from build123d import *

# Parameters (mm, degrees)
SKETCH1_W           = 10
SKETCH1_H           = 26.532998322
SKETCH1_R           = 2.25
SKETCH1_R_2         = 1.75
BOSS_EXTRUDE1_DEPTH = 4
SKETCH6_W           = 12
SKETCH6_H           = 6
BOSS_EXTRUDE3_DEPTH = 3.5
FILLET1_R           = 2
FILLET2_R           = 2
FILLET3_R           = 0.5
FILLET4_R           = 2


with BuildPart() as part:
    # Sketch1 → Boss-Extrude1 (new body)
    with BuildSketch(Plane.XY):
        with Locations((38, 0)):
            Rectangle(SKETCH1_W, SKETCH1_H)
        with Locations((38, 0)):
            Circle(SKETCH1_R, mode=Mode.SUBTRACT)
        with Locations((38, 10)):
            Circle(SKETCH1_R_2, mode=Mode.SUBTRACT)
        with Locations(Location((38, -10, 0), (0, 0, 180))):
            Circle(SKETCH1_R_2, mode=Mode.SUBTRACT)
    extrude(amount=BOSS_EXTRUDE1_DEPTH)

    # Sketch6 → Boss-Extrude3 (add)
    with BuildSketch(Plane.XY):
        with Locations((49, 0)):
            Rectangle(SKETCH6_W, SKETCH6_H)
    extrude(amount=BOSS_EXTRUDE3_DEPTH)

    # Fillet1
    fillet1_edges = [part.edges().sort_by_distance(p)[0] for p in [
        (55, -3, 1.75),
        (55, 3, 1.75),
    ]]
    fillet(fillet1_edges, radius=FILLET1_R)

    # Fillet2
    fillet2_edges = [part.edges().sort_by_distance(p)[0] for p in [
        (43, 3, 1.75),
        (43, -3, 1.75),
    ]]
    fillet(fillet2_edges, radius=FILLET2_R)

    # Fillet3
    fillet3_edges = [part.edges().sort_by_distance(p)[0] for p in [
        (43, 0, 3.5),
    ]]
    fillet(fillet3_edges, radius=FILLET3_R - 0.0001)  # a hair under: the kernel refuses the full size

    # Fillet4
    fillet4_edges = [part.edges().sort_by_distance(p)[0] for p in [
        (43, -13.266499161, 2),
        (33, -13.266499161, 2),
        (33, 13.266499161, 2),
        (43, 13.266499161, 2),
    ]]
    fillet(fillet4_edges, radius=FILLET4_R)


solid = part.part
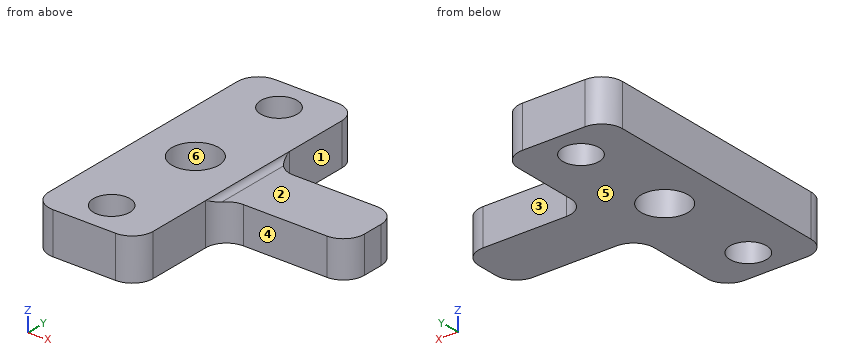
Check sheet for the modelled part. Datum: model origin and axes. Units: mm. Face numbers are marked on the shaded views. A direction names the side the tool comes from. Give positions to 0.01 mm unless a question says otherwise; leave off trailing zeros. Loops run counter-clockwise (first coordinate to the right, second up) from the corner with the lowest first, then second, coordinate; pieces in that order, holes last. Notation, with made-up numbers: M 33,14 L 81,14 A28 ccw 81,47 Z; hole C 34,9.5 d1. An arc over 180 degrees is marked long. Use a Markdown table: item, result. Add a question column.
Q1. Sectioned sample at C-C, the plane z = 1.15. Record the cut outline in (x, y), then the cut area to 3 significant figures.
Q2. Tool access check on the marked faces 1, 2 and 3. Record the directions out of +Z, -Z, +X, -X, +Y, -Y that give a thin tool (end or side, any length) a straight path to the whole face; none if there is none.
Q3. Sectioned sample at B-B, the plane y = -10. Record the cut outline in (x, z).
Q4. Scan lines: line 1 along Y through (x, z) = (38, 2.6); line 2 along X through (y, z) = (-10, 2.95); line 3 along Y through (x, z) = (52.5, 2.55). Record each from-to range of solid material in increasing order. Write a range as [from, to].
Q5. Mould release check, pull along Y, two halves, no side actions. Record for the marked faces 4, 5 and 6: pulls with the +Y half, pulls with the -Y half, needs draft (parallel to the pull), parting line crosses it, or undercut.
Q6. Sectioned sample at A-A, the plane x = 38. Record the cut outline in (y, z), then the cut area to 3 significant figures.
Q7. Sectioned sample at D-D, the plane x = 50.25. Record the cut outline in (y, z), then the cut area to 3 significant figures.
Q8. Go/stop test with flat-tipped pins: pin 1 (3 mm diameter, centred on x = 38, y = -10, fed in from -Z); pin 2 (8 mm diameter, centred on x = 48, y = 1.5, fed in from +Z); pin 3 (1.8 mm diameter, centred on x = 48, z = 1.5, fed in from -Y); pin 4 (8 mm diameter, centred on x = 46.5, y = 10, fed in from -Z). Record where each tip stops, or that it passes through.
Verdict:
| question | item | result |
|---|---|---|
| 1 | outline | M 33,-11.27 A2 ccw 35,-13.27 L 41,-13.27 A2 ccw 43,-11.27 L 43,-5 A2 cw 45,-3 L 53,-3 A2 ccw 55,-1 L 55,1 A2 ccw 53,3 L 45,3 A2 cw 43,5 L 43,11.27 A2 ccw 41,13.27 L 35,13.27 A2 ccw 33,11.27 Z; hole C 38,0 d4.5; hole C 38,-10 d3.5; hole C 38,10 d3.5 |
| 1 | area | 299 mm^2 |
| 2 | face 1 | +Z, -Z, +X |
| 2 | face 2 | +Z, +X, +Y, -Y |
| 2 | face 3 | +Z, -Z, +X, +Y |
| 3 | outline | M 33,0 L 36.25,0 L 36.25,4 L 33,4 Z; M 39.75,0 L 43,0 L 43,4 L 39.75,4 Z |
| 4 | line 1 | [-13.27, -11.75], [-8.25, -2.25], [2.25, 8.25], [11.75, 13.27] |
| 4 | line 2 | [33, 36.25], [39.75, 43] |
| 4 | line 3 | [-3, 3] |
| 5 | face 4 | pulls with the -Y half |
| 5 | face 5 | needs draft |
| 5 | face 6 | undercut |
| 6 | outline | M -13.27,0 L -11.75,0 L -11.75,4 L -13.27,4 Z; M -8.25,0 L -2.25,0 L -2.25,4 L -8.25,4 Z; M 2.25,0 L 8.25,0 L 8.25,4 L 2.25,4 Z; M 11.75,0 L 13.27,0 L 13.27,4 L 11.75,4 Z |
| 6 | area | 60.1 mm^2 |
| 7 | outline | M -3,0 L 3,0 L 3,3.5 L -3,3.5 Z |
| 7 | area | 21.0 mm^2 |
| 8 | pin 1 | through |
| 8 | pin 2 | z = 3.5 |
| 8 | pin 3 | y = -3 |
| 8 | pin 4 | z = 0 |
